Can you work these out from the model? Positions are in its coordinate system, mm. A direction names the side the tool comes from. Coordinates: 2 decimals unless noted, no trailing zeros. Order: outer loops, then holes, each group sorted by start corner. A loop starts at its lowest first (then second) coordinate and runs counter-clockwise, first axis right, second up. Notation, with made-up numbers: (32.5, 23) -> (62.5, 23) arc R12 cw to (62.5, 31) -> close; hole circle Ø11 at (27, -27.75). An arc over 180 degrees is marked (long way). Use a Markdown table: item, result. Add a question column.
1. Suppose I cut it at C-C, the plane y = 31. List the corners of the cut face in (x, z) for me, then the cut area to 3 significant figures.
2. We'd pull the mould along Y, two halves only. Please class faces 1 (the cylindrical face through (67, 14, 2)), 2 (the flat face through (57, 30, 8)), 3 (the flat face through (61, 45, 4)): pulls with the +Y half, pulls with the -Y half, needs draft (parallel to the pull), parting line crosses it, or undercut.
3. Suppose I cut it at B-B, the plane z = 6.75. List the corners of the cut face in (x, y) for me.
4. For faces 4 (the flat face through (0, 18, 4)), 5 (the cylindrical face through (89.43, 9.86, 4.45)), 6 (the cylindrical face through (90, 37.8, 4.1)), 7 (the flat face through (71, 20, 3)), which set-ups out of +Z, -Z, +X, -X, +Y, -Y let a thin tool reach every point of the face, with its end or its side?
5. If I drill on line 1 along X through (y, z) = (3.5, 4.25); line 2 along X through (y, z) = (57, 3.75); line 3 along Z through (x, y) = (6, 10.25), over which ranges is the centre line in solid material (lowest first)? Write a range as from..to.
6. Suppose I cut it at D-D, the plane x = 85. List the corners of the cut face in (y, z) for me.
7. For pin 1 Ø12.5 at (x, y) = (20.5, 18) entering from +Z; pin 2 Ø3 at (y, z) = (39.5, 2) entering from -X; pin 3 Ø0.9 at (x, z) = (6.5, 4) entering from -Y, each with a flat end and sliding along its axis, tell me the tip position at first contact or that it passes through.
8. Suppose I cut it at A-A, the plane x = 56. List the corners of the cut face in (y, z) for me.
```python
from build123d import *

# Parameters (mm, degrees)
ESQUISSE1_W             = 114.432989691
ESQUISSE1_H             = 75
BOSS_EXTRU_1_DEPTH      = 8
ESQUISSE2_R             = 7.95
ENL_V_MAT_EXTRU_1_DEPTH = 5
ENL_V_MAT_EXTRU_2_REACH = 5
ESQUISSE3_R             = 6
ENL_V_MAT_EXTRU_3_DEPTH = 9
ESQUISSE5_W             = 20.432989691
ESQUISSE5_H             = 75
ENL_V_MAT_EXTRU_4_DEPTH = 9
ENL_V_MAT_EXTRU_5_DEPTH = 9
ESQUISSE7_W             = 52
ESQUISSE7_H             = 23
ENL_V_MAT_EXTRU_6_DEPTH = 9
ESQUISSE10_R            = 1.5
ENL_V_MAT_EXTRU_7_DEPTH = 30
CONG_1_R                = 15
ESQUISSE11_R            = 1.5
ENL_V_MAT_EXTRU_8_DEPTH = 20


with BuildPart() as part:
    # Esquisse1 → Boss.-Extru.1 (new body)
    with BuildSketch(Plane.XY):
        with Locations((57.216494846, 37.5)):
            Rectangle(ESQUISSE1_W, ESQUISSE1_H)
    extrude(amount=BOSS_EXTRU_1_DEPTH)

    # Esquisse2 → Enlèv. mat.-Extru.1 (cut)
    with BuildSketch(Plane.XY.offset(8)):
        with Locations((20, 18)):
            Circle(ESQUISSE2_R)
        with Locations((73, 14)):
            Circle(ESQUISSE2_R)
    extrude(amount=-ENL_V_MAT_EXTRU_1_DEPTH, mode=Mode.SUBTRACT)

    # Esquisse3 → Enlèv. mat.-Extru.2 (cut, up to next)
    with BuildSketch(Plane.XY.offset(3), mode=Mode.PRIVATE) as enl_v_mat_extru_2_sk1:
        with Locations((20, 18)):
            Circle(ESQUISSE3_R)
    enl_v_mat_extru_2_tool1 = extrude(enl_v_mat_extru_2_sk1.sketch, amount=-ENL_V_MAT_EXTRU_2_REACH, mode=Mode.PRIVATE) & part.part
    add(enl_v_mat_extru_2_tool1.solids().sort_by_distance((20, 18, 3))[0], mode=Mode.SUBTRACT)
    # Esquisse3 → Enlèv. mat.-Extru.2 (cut, up to next)
    with BuildSketch(Plane.XY.offset(3), mode=Mode.PRIVATE) as enl_v_mat_extru_2_sk2:
        with Locations((73, 14)):
            Circle(ESQUISSE3_R)
    enl_v_mat_extru_2_tool2 = extrude(enl_v_mat_extru_2_sk2.sketch, amount=-ENL_V_MAT_EXTRU_2_REACH, mode=Mode.PRIVATE) & part.part
    add(enl_v_mat_extru_2_tool2.solids().sort_by_distance((73, 14, 3))[0], mode=Mode.SUBTRACT)

    # Esquisse4 → Enlèv. mat.-Extru.3 (cut, through all)
    with BuildSketch(Plane.XY.offset(8)):
        with BuildLine():
            ThreePointArc((50.413505675, 15.704641081), (45.525982293, 34.69353851), (30.088740957, 46.783107996))
            ThreePointArc((30.088740957, 46.783107996), (26.90252383, 45.250782829), (28.434848997, 42.064565701))
            ThreePointArc((28.434848997, 42.064565701), (41.341395032, 31.956892853), (45.427685072, 16.080929428))
            ThreePointArc((45.427685072, 16.080929428), (47.7324512, 13.399874954), (50.413505675, 15.704641081))
        make_face()
    extrude(amount=-ENL_V_MAT_EXTRU_3_DEPTH, mode=Mode.SUBTRACT)

    # Esquisse5 → Enlèv. mat.-Extru.4 (cut, through all)
    with BuildSketch(Plane.XY.offset(8)):
        with Locations((104.216494845, 37.5)):
            Rectangle(ESQUISSE5_W, ESQUISSE5_H)
    extrude(amount=-ENL_V_MAT_EXTRU_4_DEPTH, mode=Mode.SUBTRACT)

    # Esquisse6 → Enlèv. mat.-Extru.5 (cut, through all)
    with BuildSketch(Plane.XY.offset(8)):
        with BuildLine():
            Line((87.8, 40), (87.8, 47))
            ThreePointArc((87.8, 47), (90, 49.2), (92.2, 47))
            Line((92.2, 47), (92.2, 40))
            ThreePointArc((92.2, 40), (90, 37.8), (87.8, 40))
        make_face()
        with BuildLine():
            Line((58.2, 40), (58.2, 47))
            ThreePointArc((58.2, 47), (56, 49.2), (53.8, 47))
            Line((53.8, 47), (53.8, 40))
            ThreePointArc((53.8, 40), (56, 37.8), (58.2, 40))
        make_face()
    extrude(amount=-ENL_V_MAT_EXTRU_5_DEPTH, mode=Mode.SUBTRACT)

    # Esquisse7 → Enlèv. mat.-Extru.6 (cut, through all)
    with BuildSketch(Plane.XY.offset(8)):
        with Locations((26, 63.5)):
            Rectangle(ESQUISSE7_W, ESQUISSE7_H)
    extrude(amount=-ENL_V_MAT_EXTRU_6_DEPTH, mode=Mode.SUBTRACT)

    # Esquisse10 → Enlèv. mat.-Extru.7 (cut)
    with BuildSketch(Plane(origin=(0, 75, 0), x_dir=(1, 0, 0), z_dir=(0, 1, 0))):
        with Locations((85, -4)):
            Circle(ESQUISSE10_R)
        with Locations((61, -4)):
            Circle(ESQUISSE10_R)
    extrude(amount=-ENL_V_MAT_EXTRU_7_DEPTH, mode=Mode.SUBTRACT)

    # Congé1
    cong_1_edges = [part.edges().sort_by_distance(p)[0] for p in [
        (52, 52, 4),
        (0, 52, 4),
    ]]
    fillet(cong_1_edges, radius=CONG_1_R)

    # Esquisse11 → Enlèv. mat.-Extru.8 (cut)
    with BuildSketch(Plane.XZ):
        with Locations((6, 4)):
            Circle(ESQUISSE11_R)
        with Locations((88, 4)):
            Circle(ESQUISSE11_R)
    extrude(amount=-ENL_V_MAT_EXTRU_8_DEPTH, mode=Mode.SUBTRACT)


solid = part.part
```
Worked out:
| question | item | result |
|---|---|---|
| 1 | outline | (0, 0) -> (41.94, 0) -> (41.94, 8) -> (0, 8) -> close; (47.59, 0) -> (94, 0) -> (94, 8) -> (47.59, 8) -> close |
| 1 | area | 707 mm² |
| 2 | face 1 | undercut |
| 2 | face 2 | needs draft |
| 2 | face 3 | pulls with the +Y half |
| 3 | outline | (0, 0) -> (94, 0) -> (94, 75) -> (52, 75) -> (52, 67) arc R15 cw to (37, 52) -> (15, 52) arc R15 ccw to (0, 37) -> close; hole circle Ø15.9 at (20, 18); hole (28.43, 42.06) arc R25.5 cw to (45.43, 16.08) arc R2.5 ccw to (50.41, 15.7) arc R30.5 ccw to (30.09, 46.78) arc R2.5 ccw to start; hole (53.8, 40) arc R2.2 ccw to (58.2, 40) -> (58.2, 47) arc R2.2 ccw to (53.8, 47) -> close; hole circle Ø15.9 at (73, 14); hole (87.8, 40) arc R2.2 ccw to (92.2, 40) -> (92.2, 47) arc R2.2 ccw to (87.8, 47) -> close |
| 4 | face 4 | +Z, -Z, -X, +Y, -Y |
| 4 | face 5 | -Y |
| 4 | face 6 | +Z, -Z |
| 4 | face 7 | +Z |
| 5 | line 1 | x = 0..4.52, 7.48..86.52, 89.48..94 |
| 5 | line 2 | x = 48.18..59.52, 62.48..83.52, 86.48..94 |
| 5 | line 3 | z = 0..2.5, 5.5..8 |
| 6 | outline | (0, 0) -> (75, 0) -> (75, 2.5) -> (45, 2.5) -> (45, 5.5) -> (75, 5.5) -> (75, 8) -> (0, 8) -> close |
| 7 | pin 1 | stops at z = 3 |
| 7 | pin 2 | stops at x = 0.03 |
| 7 | pin 3 | stops at y = 20 |
| 8 | outline | (0, 0) -> (37.8, 0) -> (37.8, 8) -> (0, 8) -> close; (49.2, 0) -> (75, 0) -> (75, 8) -> (49.2, 8) -> close |
